from build123d import *

# Parameters (mm, degrees)
F0_R           = 4
F1_DEPTH       = 420
F4_D           = 2.4
F4_DEPTH       = 100
F4_CSINK_D     = 6.72
F4_CSINK_ANGLE = 90
F4_TIP         = 0.7210327428


with BuildPart() as f1:
    # F0 (on Front) → F1 (new body)
    with BuildSketch(Plane.XZ):
        Circle(F0_R)
    extrude(amount=-F1_DEPTH)

    # F4
    with Locations(Plane.XY.offset(4)):
        with Locations((0, 84), (0, 168), (0, 252), (0, 336)):
            CounterSinkHole(F4_D / 2, F4_CSINK_D / 2, depth=F4_DEPTH, counter_sink_angle=F4_CSINK_ANGLE)
            with Locations((0, 0, -(F4_DEPTH + F4_TIP / 2))):  # 118° drill point
                Cone(0, F4_D / 2, F4_TIP, mode=Mode.SUBTRACT)


solid = f1.part
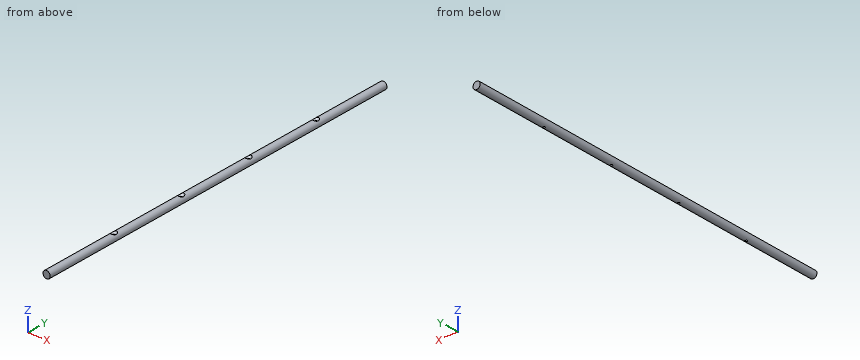
Can you work these out from the model? Positions are in its coordinate system, mm. Coordinates: 2 decimals unless noted, no trailing zeros. Write each loop counter-clockwise with the first axis right and the second up, starting at its lowest first coordinate (ties: lowest second). Pieces come first, ordered by that corner, then holes. Notation, with made-up numbers: (37, 76) -> (80, 76) arc R8 cw to (80, 80) -> close; hole circle Ø7 at (68.5, 76.25). An arc over 180 degrees is marked (long way). Write item = value, one per line.
(1) Imagine slicing it at A-A (y = 114). Please give me the cut outline in (x, z).
Verdict:
outline = circle Ø8 at (0, 0)
(2) If I drill on probe 1 along Y at (x, z) = (0, 0.3); probe 2 along Y at (x, z) = (-0.75, -0.25); probe 3 along X at (y, z) = (252, 0.2) (3 decimals), over which ranges is the centre line in solid material (lowest first)?
Verdict:
probe_1 = 0 to 82.8, 85.2 to 166.8, 169.2 to 250.8, 253.2 to 334.8, 337.2 to 420
probe_2 = 0 to 83.06, 84.94 to 167.06, 168.94 to 251.06, 252.94 to 335.06, 336.94 to 420
probe_3 = -3.995 to -1.2, 1.2 to 3.995
(3) For pin 1 (1 mm diameter, centred on x = 1.5, y = 206.5, fed in from -Z); pin 2 (3 mm diameter, centred on y = 167.5, z = 2, fed in from -X); pin 3 (3 mm diameter, centred on x = 0, y = 84, fed in from +Z); pin 4 (1.9 mm diameter, centred on x = 0, y = 168, fed in from -Z), each with a flat end and sliding along its axis, tell me the tip position at first contact or that it passes through.
Verdict:
pin_1 = -3.87
pin_2 = -3.97
pin_3 = 2.14
pin_4 = through
